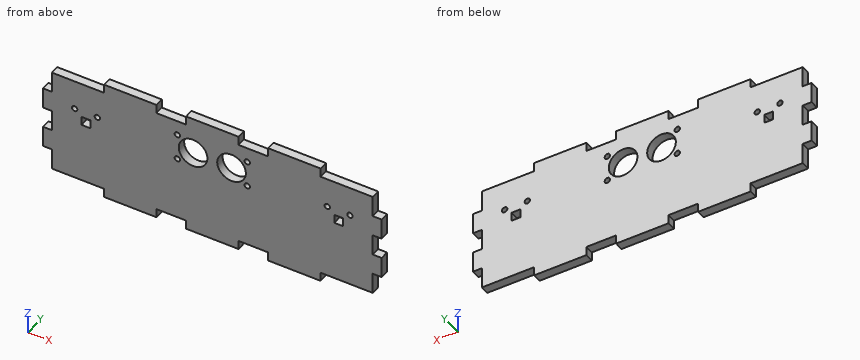
```python
from build123d import *

# Parameters (mm, degrees)
SKETCH1_R           = 8.2
SKETCH1_R_2         = 1.55
SKETCH1_W           = 5
SKETCH1_H           = 5
BOSS_EXTRUDE1_DEPTH = 5


with BuildPart() as part:
    # Sketch1 → Boss-Extrude1 (new body)
    with BuildSketch(Plane(origin=(0, 0, 0), x_dir=(1, 0, 0), z_dir=(0, 1, 0))):
        Polygon((-87.414457831, -48), (-57.614457831, -48), (-57.614457831, -53.1), (-27.614457831, -53.1), (-27.614457831, -48), (-10.614457831, -48), (-10.614457831, -53.1), (19.385542169, -53.1), (19.385542169, -48), (36.385542169, -48), (36.385542169, -53.1), (66.385542169, -53.1), (66.385542169, -48), (96.185542169, -48), (96.185542169, -36), (101.285542169, -36), (101.285542169, -24), (96.185542169, -24), (96.185542169, -12), (101.285542169, -12), (101.285542169, 0), (96.185542169, 0), (96.185542169, 12), (66.385542169, 12), (66.385542169, 17.1), (36.385542169, 17.1), (36.385542169, 12), (19.385542169, 12), (19.385542169, 17.1), (-10.614457831, 17.1), (-10.614457831, 12), (-27.614457831, 12), (-27.614457831, 17.1), (-57.614457831, 17.1), (-57.614457831, 12), (-87.414457831, 12), (-87.414457831, 0), (-92.514457831, 0), (-92.514457831, -12), (-87.414457831, -12), (-87.414457831, -24), (-92.514457831, -24), (-92.514457831, -36), (-87.414457831, -36), align=None)
        with Locations(Location((15.385542169, -32, 0), (0, 0, 270))):
            Circle(SKETCH1_R, mode=Mode.SUBTRACT)
        with Locations(Location((-6.614457831, -32, 0), (0, 0, 90))):
            Circle(SKETCH1_R, mode=Mode.SUBTRACT)
        with Locations(Location((-15.614457831, -24.5, 0), (0, 0, 270))):
            Circle(SKETCH1_R_2, mode=Mode.SUBTRACT)
        with Locations(Location((-15.614457831, -39.5, 0), (0, 0, 270))):
            Circle(SKETCH1_R_2, mode=Mode.SUBTRACT)
        with Locations(Location((-74.414457831, -31, 0), (0, 0, 270))):
            Circle(SKETCH1_R_2, mode=Mode.SUBTRACT)
        with Locations(Location((-61.414457831, -31, 0), (0, 0, 270))):
            Circle(SKETCH1_R_2, mode=Mode.SUBTRACT)
        with Locations(Location((24.385542169, -39.5, 0), (0, 0, 90))):
            Circle(SKETCH1_R_2, mode=Mode.SUBTRACT)
        with Locations(Location((24.385542169, -24.5, 0), (0, 0, 90))):
            Circle(SKETCH1_R_2, mode=Mode.SUBTRACT)
        with Locations(Location((70.185542169, -31, 0), (0, 0, 90))):
            Circle(SKETCH1_R_2, mode=Mode.SUBTRACT)
        with Locations(Location((83.185542169, -31, 0), (0, 0, 90))):
            Circle(SKETCH1_R_2, mode=Mode.SUBTRACT)
        with Locations((-67.914457831, -25)):
            Rectangle(SKETCH1_W, SKETCH1_H, mode=Mode.SUBTRACT)
        with Locations((76.685542169, -25)):
            Rectangle(SKETCH1_W, SKETCH1_H, mode=Mode.SUBTRACT)
    extrude(amount=BOSS_EXTRUDE1_DEPTH)


solid = part.part
```
Can you work these out from the model? Positions are in its coordinate system, mm. Give positions to 0.01 mm unless a question says otherwise; leave off trailing zeros. Order: outer loops, then holes, each group sorted by start corner. A loop starts at its lowest first (then second) coordinate and runs counter-clockwise, first axis right, second up. Notation, with made-up numbers: (-15, -40) - (23, -40) arc R28 cw to (23, -6) - close; hole circle Ø5 at (12, 45.25). An arc over 180 degrees is marked (long way). Use a Markdown table: item, result. Add a question column.
Q1. If we section it at A-A on x = 32: Write out the boundary of the cut face in (y, z), plus the area to 3 significant figures.
Q2. If we section it at B-B on z = -8: Write out the boundary of the cut face in (x, y), plus the area to 3 significant figures.
Q3. If we section it at C-C on y = 3: Count the separate pieces of the cut face and the enclosed holes in it, plus the area to 3 significant figures.
Q4. I'm going to push flat-ended pins straight in: pin 1 (1.5 mm diameter, centred on x = -90.5, y = 2, fed in from +Z); pin 2 (2.5 mm diameter, centred on x = 99.5, y = 1.5, fed in from -Z); pin 3 (1.5 mm diameter, centred on y = 3.5, z = 43, fed in from +X). Where does each tip first touch, or does it pass through?
Q5. Please list where these lines run through material, in increasing order: line 1 along X through (y, z) = (3.4, 39.5); line 2 along X through (y, z) = (1.9, 37.5); line 3 along Z through (x, y) = (32, 3.7).
Answers follow:
| question | item | result |
|---|---|---|
| 1 | outline | (0, -12) - (5, -12) - (5, 48) - (0, 48) - close |
| 1 | area | 300 mm^2 |
| 2 | outline | (-87.41, 0) - (96.19, 0) - (96.19, 5) - (-87.41, 5) - close |
| 2 | area | 918 mm^2 |
| 3 | separate pieces | 1 |
| 3 | enclosed holes | 12 |
| 3 | area | 11,600 mm^2 |
| 4 | pin 1 | stops at z = 36 |
| 4 | pin 2 | stops at z = 0 |
| 4 | pin 3 | stops at x = 96.19 |
| 5 | line 1 | x = -87.41 to -17.16, -14.06 to -9.93, -3.3 to 12.07, 18.7 to 22.84, 25.94 to 96.19 |
| 5 | line 2 | x = -87.41 to -12.7, -0.53 to 9.3, 21.47 to 96.19 |
| 5 | line 3 | z = -12 to 48 |
